from build123d import *

# Parameters (mm, degrees)
SKETCH_1_W          = 114
SKETCH_1_H          = 68
EXTRUDE_1_DEPTH     = 1
CUT_EXTRUDE_1_REACH = 3
SKETCH_2_R          = 2.25


with BuildPart() as part:
    # Эскиз1 → Бобышка-Вытянуть1 (new body)
    with BuildSketch(Plane.XY):
        with Locations((57, 34)):
            Rectangle(SKETCH_1_W, SKETCH_1_H)
    extrude(amount=EXTRUDE_1_DEPTH)

    # Эскиз2 → Вырез-Вытянуть1 (cut, up to next)
    with BuildSketch(Plane.XY.offset(1), mode=Mode.PRIVATE) as cut_extrude_1_sk1:
        with Locations((6, 62)):
            Circle(SKETCH_2_R)
    cut_extrude_1_tool1 = extrude(cut_extrude_1_sk1.sketch, amount=-CUT_EXTRUDE_1_REACH, mode=Mode.PRIVATE) & part.part
    add(cut_extrude_1_tool1.solids().sort_by_distance((6, 62, 1))[0], mode=Mode.SUBTRACT)
    # Эскиз2 → Вырез-Вытянуть1 (cut, up to next)
    with BuildSketch(Plane.XY.offset(1), mode=Mode.PRIVATE) as cut_extrude_1_sk2:
        with Locations((6, 28)):
            Circle(SKETCH_2_R)
    cut_extrude_1_tool2 = extrude(cut_extrude_1_sk2.sketch, amount=-CUT_EXTRUDE_1_REACH, mode=Mode.PRIVATE) & part.part
    add(cut_extrude_1_tool2.solids().sort_by_distance((6, 28, 1))[0], mode=Mode.SUBTRACT)
    # Эскиз2 → Вырез-Вытянуть1 (cut, up to next)
    with BuildSketch(Plane.XY.offset(1), mode=Mode.PRIVATE) as cut_extrude_1_sk3:
        with Locations((6, 6)):
            Circle(SKETCH_2_R)
    cut_extrude_1_tool3 = extrude(cut_extrude_1_sk3.sketch, amount=-CUT_EXTRUDE_1_REACH, mode=Mode.PRIVATE) & part.part
    add(cut_extrude_1_tool3.solids().sort_by_distance((6, 6, 1))[0], mode=Mode.SUBTRACT)
    # Эскиз2 → Вырез-Вытянуть1 (cut, up to next)
    with BuildSketch(Plane.XY.offset(1), mode=Mode.PRIVATE) as cut_extrude_1_sk4:
        with Locations((57, 6)):
            Circle(SKETCH_2_R)
    cut_extrude_1_tool4 = extrude(cut_extrude_1_sk4.sketch, amount=-CUT_EXTRUDE_1_REACH, mode=Mode.PRIVATE) & part.part
    add(cut_extrude_1_tool4.solids().sort_by_distance((57, 6, 1))[0], mode=Mode.SUBTRACT)
    # Эскиз2 → Вырез-Вытянуть1 (cut, up to next)
    with BuildSketch(Plane.XY.offset(1), mode=Mode.PRIVATE) as cut_extrude_1_sk5:
        with Locations((57, 62)):
            Circle(SKETCH_2_R)
    cut_extrude_1_tool5 = extrude(cut_extrude_1_sk5.sketch, amount=-CUT_EXTRUDE_1_REACH, mode=Mode.PRIVATE) & part.part
    add(cut_extrude_1_tool5.solids().sort_by_distance((57, 62, 1))[0], mode=Mode.SUBTRACT)
    # Эскиз2 → Вырез-Вытянуть1 (cut, up to next)
    with BuildSketch(Plane.XY.offset(1), mode=Mode.PRIVATE) as cut_extrude_1_sk6:
        with Locations((108, 62)):
            Circle(SKETCH_2_R)
    cut_extrude_1_tool6 = extrude(cut_extrude_1_sk6.sketch, amount=-CUT_EXTRUDE_1_REACH, mode=Mode.PRIVATE) & part.part
    add(cut_extrude_1_tool6.solids().sort_by_distance((108, 62, 1))[0], mode=Mode.SUBTRACT)
    # Эскиз2 → Вырез-Вытянуть1 (cut, up to next)
    with BuildSketch(Plane.XY.offset(1), mode=Mode.PRIVATE) as cut_extrude_1_sk7:
        with Locations((108, 28)):
            Circle(SKETCH_2_R)
    cut_extrude_1_tool7 = extrude(cut_extrude_1_sk7.sketch, amount=-CUT_EXTRUDE_1_REACH, mode=Mode.PRIVATE) & part.part
    add(cut_extrude_1_tool7.solids().sort_by_distance((108, 28, 1))[0], mode=Mode.SUBTRACT)
    # Эскиз2 → Вырез-Вытянуть1 (cut, up to next)
    with BuildSketch(Plane.XY.offset(1), mode=Mode.PRIVATE) as cut_extrude_1_sk8:
        with Locations((108, 6)):
            Circle(SKETCH_2_R)
    cut_extrude_1_tool8 = extrude(cut_extrude_1_sk8.sketch, amount=-CUT_EXTRUDE_1_REACH, mode=Mode.PRIVATE) & part.part
    add(cut_extrude_1_tool8.solids().sort_by_distance((108, 6, 1))[0], mode=Mode.SUBTRACT)


solid = part.part
Read the model definition and answer for the solid it produces. Units are mm, in the model's axes. Round coordinates to 2 decimals unless told otherwise and drop trailing zeros. Write each loop counter-clockwise with the first axis right and the second up, starting at its lowest first coordinate (ties: lowest second). Pieces come first, ordered by that corner, then holes.
1. The part is cut by section A-A, the plane y = 28. Determine the outline of the cut face in (x, z).
2. Determine the mould class of faces 1 (the face through (54.752, 6.099, 0.507)), 2 (the face through (56, 34, 1)) for opening direction Y: pulls with the +Y half, pulls with the -Y half, needs draft (parallel to the pull), parting line crosses it, or undercut.
3. The part is cut by section D-D, the plane x = 57. Determine the outline of the cut face in (y, z), then the cut area to 3 significant figures.
4. The part is cut by section C-C, the plane y = 6. Determine the outline of the cut face in (x, z), then the cut area to 4 significant figures.
5. The part is cut by section B-B, the plane z = 0.15. State how many separate pieces and enclosed holes the cut face has, then the cut area to 3 significant figures.
6. Straight lines are drawn through the part: L1, parallel to Y at x = 108, z = 0.7; L2, parallel to X at y = 63.5, z = 0.15; L3, parallel to X at y = 28.5, z = 0.1. For each, find the intervals that lie inside material, in ascending order.
Values:
1. outline: (0, 0) - (3.75, 0) - (3.75, 1) - (0, 1) - close; (8.25, 0) - (105.75, 0) - (105.75, 1) - (8.25, 1) - close; (110.25, 0) - (114, 0) - (114, 1) - (110.25, 1) - close
2. face 1: undercut
2. face 2: needs draft
3. outline: (0, 0) - (3.75, 0) - (3.75, 1) - (0, 1) - close; (8.25, 0) - (59.75, 0) - (59.75, 1) - (8.25, 1) - close; (64.25, 0) - (68, 0) - (68, 1) - (64.25, 1) - close
3. area: 59.0 mm2
4. outline: (0, 0) - (3.75, 0) - (3.75, 1) - (0, 1) - close; (8.25, 0) - (54.75, 0) - (54.75, 1) - (8.25, 1) - close; (59.25, 0) - (105.75, 0) - (105.75, 1) - (59.25, 1) - close; (110.25, 0) - (114, 0) - (114, 1) - (110.25, 1) - close
4. area: 100.5 mm2
5. separate pieces: 1
5. enclosed holes: 8
5. area: 7,620 mm2
6. L1: y = 0 to 3.75, 8.25 to 25.75, 30.25 to 59.75, 64.25 to 68
6. L2: x = 0 to 4.32, 7.68 to 55.32, 58.68 to 106.32, 109.68 to 114
6. L3: x = 0 to 3.81, 8.19 to 105.81, 110.19 to 114
